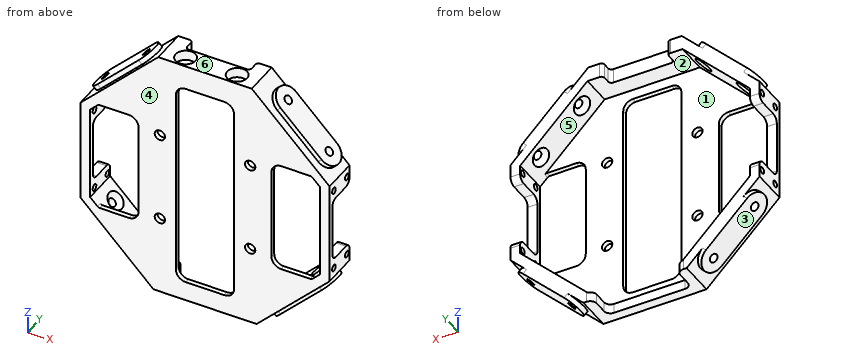
from build123d import *

# Parameters (mm, degrees)
BOSS_EXTRUDE1_DEPTH                        = 11
SHELL1_T                                   = -3
SHELL1_THICKNESS_2_DEPTH                   = 1.5
SKETCH2_R                                  = 1.3
CUT_EXTRUDE1_DEPTH                         = 152
SKETCH3_R                                  = 1.3
CUT_EXTRUDE2_DEPTH                         = 152
CUT_EXTRUDE3_DEPTH                         = 152
SKETCH5_W                                  = 13
SKETCH5_H                                  = 8
CUT_EXTRUDE4_DEPTH                         = 45
FILLET1_R                                  = 2
CUT_EXTRUDE6_DEPTH                         = 92
SKETCH6_R                                  = 1
CUT_EXTRUDE7_DEPTH                         = 5
SKETCH12_R                                 = 1
CUT_EXTRUDE8_DEPTH                         = 5
FILLET2_R                                  = 1
BOSS_EXTRUDE2_DEPTH                        = 11
SKETCH14_R                                 = 3.1
CUT_EXTRUDE9_DEPTH                         = 3.1
CUT_EXTRUDE10_DEPTH                        = 9.1
FILLET3_R                                  = 1
SKETCH19_R                                 = 1.6
CUT_EXTRUDE12_DEPTH                        = 10
FILLET4_R                                  = 3
CHAMFER1_SIZE                              = 1.5
BOSS_EXTRUDE3_START                        = 1.5
SKETCH20_R                                 = 1.3
BOSS_EXTRUDE3_DEPTH                        = 1.5
MIRROR1_START                              = 1.5
MIRROR1_AT_THE_SECOND_PLANE_COPY_1_SKETC_R = 1.3
MIRROR1_AT_THE_SECOND_PLANE_COPY_1_DEPTH   = 1.5


with BuildPart() as part:
    # Sketch1 → Boss-Extrude1 (new body)
    with BuildSketch(Plane(origin=(0, 0, 0), x_dir=(1, 0, 0), z_dir=(0, 1, 0))):
        Polygon((38.627416998, 16), (16, 38.627416998), (-16, 38.627416998), (-38.627416998, 16), (-38.627416998, -16), (-16, -38.627416998), (16, -38.627416998), (38.627416998, -16), align=None)
    extrude(amount=BOSS_EXTRUDE1_DEPTH)

    # Shell1
    shell1_openings = [part.faces().sort_by_distance(p)[0] for p in [
        (0, 11, 0),
    ]]
    offset(amount=SHELL1_T, openings=shell1_openings, kind=Kind.INTERSECTION)

    # Shell1 thickness 2 face (on inner face of the shell) → Shell1 thickness 2 (cut)
    with BuildSketch(Plane(origin=(0, 3, 0), x_dir=(0, 0, -1), z_dir=(0, -1, 0))):
        Polygon((-14.757359313, 35.627416998), (14.757359313, 35.627416998), (35.627416998, 14.757359313), (35.627416998, -14.757359313), (14.757359313, -35.627416998), (-14.757359313, -35.627416998), (-35.627416998, -14.757359313), (-35.627416998, 14.757359313), align=None)
    extrude(amount=SHELL1_THICKNESS_2_DEPTH, mode=Mode.SUBTRACT)

    # Sketch2 → Cut-Extrude1 (cut)
    with BuildSketch(Plane(origin=(27.313708499, 0, 27.313708499), x_dir=(0.7071067811865475, 0, -0.7071067811865477), z_dir=(0.7071067811865477, 0, 0.7071067811865475))):
        with Locations((9, 6.75)):
            Circle(SKETCH2_R)
        with Locations((-9, 6.75)):
            Circle(SKETCH2_R)
    extrude(amount=-CUT_EXTRUDE1_DEPTH, mode=Mode.SUBTRACT)

    # Sketch3 → Cut-Extrude2 (cut)
    with BuildSketch(Plane(origin=(-27.313708499, 0, 27.313708499), x_dir=(0.7071067811865476, 0, 0.7071067811865476), z_dir=(-0.7071067811865476, 0, 0.7071067811865476))):
        with Locations((9, 6.75)):
            Circle(SKETCH3_R)
        with Locations((-9, 6.75)):
            Circle(SKETCH3_R)
    extrude(amount=-CUT_EXTRUDE2_DEPTH, mode=Mode.SUBTRACT)

    # Sketch4 → Cut-Extrude3 (cut)
    with BuildSketch(Plane(origin=(38.627416998, 0, 0), x_dir=(0, 0, -1), z_dir=(1, 0, 0))):
        Polygon((0, 1.5), (10, 1.5), (10, 11), (0, 11), (-10, 11), (-10, 1.5), align=None)
    extrude(amount=-CUT_EXTRUDE3_DEPTH, mode=Mode.SUBTRACT)

    # Sketch5 → Cut-Extrude4 (cut)
    with BuildSketch(Plane(origin=(0, 0, -38.627416998), x_dir=(-1, 0, 0), z_dir=(0, 0, -1))):
        with Locations((-6.5, 7)):
            Rectangle(SKETCH5_W, SKETCH5_H)
        with Locations((6.5, 7)):
            Rectangle(SKETCH5_W, SKETCH5_H)
    extrude(amount=-CUT_EXTRUDE4_DEPTH, mode=Mode.SUBTRACT)

    # Fillet1
    fillet1_edges = [part.edges().sort_by_distance(p)[0] for p in [
        (-13, 11, -37.127416998),
        (-13, 3, -37.127416998),
        (13, 11, -37.127416998),
        (13, 3, -37.127416998),
        (37.127416998, 11, 10),
        (37.127416998, 1.5, 10),
        (37.127416998, 11, -10),
        (37.127416998, 1.5, -10),
        (-37.127416998, 11, -10),
        (-37.127416998, 1.5, -10),
        (-37.127416998, 11, 10),
        (-37.127416998, 1.5, 10),
    ]]
    fillet(fillet1_edges, radius=FILLET1_R)

    # Sketch7 → Cut-Extrude6 (cut)
    with BuildSketch(Plane(origin=(0, 1.5, 0), x_dir=(1, 0, 0), z_dir=(0, 1, 0))):
        Polygon((35.627416998, -10.000000003), (31.627416998, -10.000000003), (31.627416998, -18.757359313), (35.627416998, -14.757359313), align=None)
        Polygon((35.627416998, 14.757359313), (35.627416998, 10.000000003), (31.627416998, 10.000000003), (31.627416998, 18.757359313), align=None)
        Polygon((-35.627416998, 10.000000003), (-31.627416998, 10.000000003), (-31.627416998, 18.757359313), (-35.627416998, 14.757359313), align=None)
        Polygon((-35.627416998, -14.757359313), (-35.627416998, -10.000000003), (-31.627416998, -10.000000003), (-31.627416998, -18.757359313), align=None)
    extrude(amount=-CUT_EXTRUDE6_DEPTH, mode=Mode.SUBTRACT)

    # Sketch6 → Cut-Extrude7 (cut)
    with BuildSketch(Plane(origin=(38.627416998, 0, 0), x_dir=(0, 0, -1), z_dir=(1, 0, 0))):
        with Locations((-13, 9.5)):
            Circle(SKETCH6_R)
        with Locations((-13, 2.4)):
            Circle(SKETCH6_R)
        with Locations((13, 2.4)):
            Circle(SKETCH6_R)
        with Locations((13, 9.5)):
            Circle(SKETCH6_R)
    extrude(amount=-CUT_EXTRUDE7_DEPTH, mode=Mode.SUBTRACT)

    # Sketch12 → Cut-Extrude8 (cut)
    with BuildSketch(Plane(origin=(-35.627416998, 0, 0), x_dir=(0, 0, -1), z_dir=(1, 0, 0))):
        with Locations((-13, 9.5)):
            Circle(SKETCH12_R)
        with Locations((-13, 2.4)):
            Circle(SKETCH12_R)
        with Locations((13, 2.4)):
            Circle(SKETCH12_R)
        with Locations((13, 9.5)):
            Circle(SKETCH12_R)
    extrude(amount=-CUT_EXTRUDE8_DEPTH, mode=Mode.SUBTRACT)

    # Fillet2
    fillet2_edges = [part.edges().sort_by_distance(p)[0] for p in [
        (-31.627416998, 0.75, 10.000000003),
        (-31.627416998, 0.75, 18.757359313),
        (-35.627416998, 0.75, 10.000000003),
        (35.627416998, 0.75, -10.000000003),
        (31.627416998, 0.75, -10.000000003),
        (31.627416998, 0.75, -18.757359313),
        (31.627416998, 0.75, 10.000000003),
        (35.627416998, 0.75, 10.000000003),
        (31.627416998, 0.75, 18.757359313),
        (-31.627416998, 0.75, -10.000000003),
        (-35.627416998, 0.75, -10.000000003),
        (-31.627416998, 0.75, -18.757359313),
    ]]
    fillet(fillet2_edges, radius=FILLET2_R)

    # Sketch13 → Boss-Extrude2 (add)
    with BuildSketch(Plane(origin=(0, 11, 0), x_dir=(1, 0, 0), z_dir=(0, 1, 0))):
        Polygon((0, -38.627416998), (-16, -38.627416998), (-14.5, -40.127416998), (0, -40.127416998), align=None)
        Polygon((16, -38.627416998), (0, -38.627416998), (0, -40.127416998), (14.5, -40.127416998), align=None)
    extrude(amount=-BOSS_EXTRUDE2_DEPTH)

    # Sketch14 → Cut-Extrude9 (cut)
    with BuildSketch(Plane.XY.offset(40.127416998)):
        with Locations((8, 3.5)):
            Circle(SKETCH14_R)
        with Locations((-8, 3.5)):
            Circle(SKETCH14_R)
    extrude(amount=-CUT_EXTRUDE9_DEPTH, mode=Mode.SUBTRACT)

    # Sketch18 → Cut-Extrude10 (cut)
    with BuildSketch(Plane.XY.offset(40.127416998)):
        Polygon((-10, 7), (0, 7), (10, 7), (10, 11), (-10, 11), align=None)
    extrude(amount=-CUT_EXTRUDE10_DEPTH, mode=Mode.SUBTRACT)

    # Fillet3
    fillet3_edges = [part.edges().sort_by_distance(p)[0] for p in [
        (-10, 7, 37.877416998),
        (-10, 11, 37.877416998),
        (10, 11, 37.877416998),
        (10, 7, 37.877416998),
    ]]
    fillet(fillet3_edges, radius=FILLET3_R)

    # Sketch19 → Cut-Extrude12 (cut)
    with BuildSketch(Plane(origin=(0, 0, 0), x_dir=(-1, 0, 0), z_dir=(0, -1, 0))):
        Polygon((9, -32.556349186), (9, 32.556349186), (-9, 32.556349186), (-9, -14), (-9, -32.556349186), align=None)
        with Locations(Location((-14, -14, 0), (0, 0, 90))):
            Circle(SKETCH19_R)
        Polygon((-20.627416998, -17.343145751), (-20.627416998, 17.343145751), (-32.627416998, 17.343145751), (-32.627416998, 11.000000003), (-35.627416998, 11.000000003), (-35.627416998, -11.000000003), (-32.627416998, -11), (-32.627416998, -17.343145751), align=None)
        Polygon((35.627416998, -11.000000003), (35.627416998, 11.000000003), (32.627416998, 11.000000003), (32.627416998, 17.343145751), (20.627416998, 17.343145751), (20.627416998, -17.343145751), (32.627416998, -17.343145751), (32.627416998, -11), align=None)
        with Locations(Location((14, -14, 0), (0, 0, 90))):
            Circle(SKETCH19_R)
        with Locations(Location((-14, 14, 0), (0, 0, 90))):
            Circle(SKETCH19_R)
        with Locations(Location((14, 14, 0), (0, 0, 90))):
            Circle(SKETCH19_R)
    extrude(amount=-CUT_EXTRUDE12_DEPTH, mode=Mode.SUBTRACT)

    # Fillet4
    fillet4_edges = [part.edges().sort_by_distance(p)[0] for p in [
        (-20.627416998, 0.75, 17.343145751),
        (-20.627416998, 0.75, -17.343145751),
        (20.627416998, 0.75, -17.343145751),
        (20.627416998, 0.75, 17.343145751),
        (-9, 0.75, 32.556349186),
        (9, 0.75, 32.556349186),
        (9, 0.75, -32.556349186),
        (-9, 0.75, -32.556349186),
    ]]
    fillet(fillet4_edges, radius=FILLET4_R)

    # Chamfer1
    chamfer1_edges = [part.edges().sort_by_distance(p)[0] for p in [
        (17.909188309, 6.75, 32.475588002),
        (-32.475588002, 6.75, -17.909188309),
        (30.637110371, 6.75, 19.74766594),
        (-19.74766594, 6.75, -30.637110371),
        (-19.74766594, 6.75, 30.637110371),
        (30.637110371, 6.75, -19.74766594),
        (-32.475588002, 6.75, 17.909188309),
        (17.909188309, 6.75, -32.475588002),
    ]]
    chamfer(chamfer1_edges, length=CHAMFER1_SIZE)

    # Sketch20 → Boss-Extrude3 (add)
    with BuildSketch(Plane(origin=(27.313708499, 0, 27.313708499), x_dir=(0.7071067811865475, 0, -0.7071067811865477), z_dir=(0.7071067811865477, 0, 0.7071067811865475)).offset(BOSS_EXTRUDE3_START)):
        with BuildLine():
            Line((-9, 2.5), (9, 2.5))
            ThreePointArc((9, 2.5), (13.25, 6.75), (9, 11))
            Line((9, 11), (-9, 11))
            ThreePointArc((-9, 11), (-13.25, 6.75), (-9, 2.5))
        make_face()
        with Locations((-9, 6.75)):
            Circle(SKETCH20_R, mode=Mode.SUBTRACT)
        with Locations((9, 6.75)):
            Circle(SKETCH20_R, mode=Mode.SUBTRACT)
    boss_extrude3 = extrude(amount=-BOSS_EXTRUDE3_DEPTH)

    # Mirror1: Boss-Extrude3 across plane
    add(boss_extrude3.mirror(Plane(origin=(0, 0, 0), x_dir=(0, 0, 1), z_dir=(1, 0, 0))))

    # Mirror1 at the second plane: Boss-Extrude3 across plane
    add(boss_extrude3.mirror(Plane.XY))

    # Mirror1 at the second plane copy 1 sketc → Mirror1 at the second plane copy 1 (add)
    with BuildSketch(Plane(origin=(-27.313708499, 0, -27.313708499), x_dir=(-0.7071067811865475, 0, 0.7071067811865477), z_dir=(-0.7071067811865477, 0, -0.7071067811865475)).offset(MIRROR1_START)):
        with BuildLine():
            Line((-9, 2.5), (9, 2.5))
            ThreePointArc((9, 2.5), (13.25, 6.75), (9, 11))
            Line((9, 11), (-9, 11))
            ThreePointArc((-9, 11), (-13.25, 6.75), (-9, 2.5))
        make_face()
        with Locations((-9, 6.75)):
            Circle(MIRROR1_AT_THE_SECOND_PLANE_COPY_1_SKETC_R, mode=Mode.SUBTRACT)
        with Locations((9, 6.75)):
            Circle(MIRROR1_AT_THE_SECOND_PLANE_COPY_1_SKETC_R, mode=Mode.SUBTRACT)
    extrude(amount=-MIRROR1_AT_THE_SECOND_PLANE_COPY_1_DEPTH)


solid = part.part
Here's how the part is built. I have some questions about the finished solid (model axes, mm). Face numbers are marked on the shaded views. A direction names the side the tool comes from. Round coordinates to 2 decimals unless told otherwise and drop trailing zeros. Write each loop counter-clockwise with the first axis right and the second up, starting at its lowest first coordinate (ties: lowest second). Pieces come first, ordered by that corner, then holes.
1. For the marked faces 5 and 6, which set-ups out of +Z, -Z, +X, -X, +Y, -Y let a thin tool reach every point of the face, with its end or its side?
2. Will these pins go through, and if not, where does the flat tip stop? pin 1 Ø1 at (x, y) = (-28.5, 4) entering from -Z; pin 2 Ø3.5 at (x, z) = (0.5, -36.5) entering from +Y; pin 3 Ø0.9 at (x, z) = (-37, 4) entering from +Y.
3. Suppose I cut it at B-B (x = -8). List the corners of the cut face in (y, z) for me.
4. I need wall thicknesses on L1, parallel to Y at x = -37.55, z = 13; L2, parallel to X at y = 2.25, z = -10; L3, parallel to Z at x = 14, y = 4.5. Which ranges of each line are inside material? Lowest first, please.
5. Suppose I cut it at A-A (z = 3). List the corners of the cut face in (x, y) for me.
6. If we mould it in two halves opening along Z, with no side actions, what happens to the marked faces 1, 2, 3 and 4? For each: released by +Z, released by -Z, zero draft, split by the parting line, or undercut.
Answer sheet:
1. face 5: +Y
1. face 6: +Z, +X, -X, +Y, -Y
2. pin 1: stops at z = -28.75
2. pin 2: stops at y = 3
2. pin 3: stops at y = 1.5
3. outline: (0, -38.63) - (3, -38.63) - (3, -35.63) - (1.5, -35.63) - (1.5, -31.79) - (0, -31.79) - close; (0, 31.79) - (1.5, 31.79) - (1.5, 35.63) - (7, 35.63) - (7, 40.13) - (6.6, 40.13) - (6.6, 37.03) - (0.4, 37.03) - (0.4, 40.13) - (0, 40.13) - close
4. L1: y = 0 to 1.4, 3.4 to 8.5, 10.5 to 11
4. L2: x = -38.63 to -35.63, 35.63 to 38.63
4. L3: z = -38.63 to -35.63, 35.63 to 40.13
5. outline: (-38.63, 0) - (-35.63, 0) - (-35.63, 1.5) - (-38.63, 1.5) - close; (-20.63, 0) - (-9, 0) - (-9, 1.5) - (-20.63, 1.5) - close; (9, 0) - (20.63, 0) - (20.63, 1.5) - (9, 1.5) - close; (35.63, 0) - (38.63, 0) - (38.63, 1.5) - (35.63, 1.5) - close
6. face 1: undercut
6. face 2: undercut
6. face 3: released by -Z
6. face 4: zero draft
